Input: part model. Units: mm. Frame: model coordinates. Face numbers are marked on the shaded views. A direction names the side the tool comes from. Coordinates: 2 decimals unless noted, no trailing zeros. Order: outer loops, then holes, each group sorted by start corner. A loop starts at its lowest first (then second) coordinate and runs counter-clockwise, first axis right, second up. Notation, with made-up numbers: (-11.5, -33.75) -> (34.5, -33.75) arc R21 ccw to (34.5, -4.75) -> close; hole circle Ø10 at (15.5, -38). An arc over 180 degrees is marked (long way). Write each question's results on one line, items separated by ' | '.
```python
from build123d import *

# Parameters (mm, degrees)
BOSS_EXTRUDE1_DEPTH     = 57
SKETCH3_W               = 33
SKETCH3_H               = 9
SKETCH3_W_2             = 9
SKETCH3_H_2             = 15.5
CUT_EXTRUDE2_DEPTH      = 86.030876745
FILLET1_R               = 4
CUT_EXTRUDE3_DEPTH      = 86.030876745
CUT_EXTRUDE4_REACH      = 81.789
CUT_EXTRUDE5_DEPTH      = 3.5
SKETCH9_R               = 3.2
SKETCH10_R              = 2.8
CUT_EXTRUDE6_DEPTH      = 82.124903768
CUT_EXTRUDE6_DEPTH_BACK = 82.124903768
SKETCH11_R              = 2
SKETCH13_R              = 2
CUT_EXTRUDE7_DEPTH      = 20
SKETCH14_R              = 1.75
SKETCH14_R_2            = 5.5
BOSS_EXTRUDE2_DEPTH     = 10
BOSS_EXTRUDE3_DEPTH     = 30
SKETCH16_R              = 2.1
CUT_EXTRUDE8_DEPTH      = 3.4
SKETCH18_R              = 2.1
CUT_EXTRUDE9_DEPTH      = 9


with BuildPart() as part:
    # Sketch1 → Boss-Extrude1 (new body)
    with BuildSketch(Plane.XY):
        Polygon((0, 0), (0, -35), (19, -35), (19, -16), (52.5, -16), (52.5, 0), align=None)
    extrude(amount=BOSS_EXTRUDE1_DEPTH)

    # Sketch3 → Cut-Extrude2 (cut, through all)
    with BuildSketch(Plane.ZY):
        with Locations((28.5, -8)):
            Rectangle(SKETCH3_W, SKETCH3_H)
        with Locations((52.5, -27.25)):
            Rectangle(SKETCH3_W_2, SKETCH3_H_2)
    extrude(amount=-CUT_EXTRUDE2_DEPTH, mode=Mode.SUBTRACT)

    # Fillet1
    fillet1_edges = [part.edges().sort_by_distance(p)[0] for p in [
        (26.25, 0, 57),
        (9.5, -19.5, 57),
    ]]
    fillet(fillet1_edges, radius=FILLET1_R)

    # Sketch4 → Cut-Extrude3 (cut, through all)
    with BuildSketch(Plane(origin=(0, 0, 0), x_dir=(-1, 0, 0), z_dir=(0, 0, -1))):
        with BuildLine():
            Line((-0.01301942, -25.002808416), (-2.010278489, -25.107480328))
            ThreePointArc((-2.010278489, -25.107480328), (-16.998857714, -25.369106952), (-2.028539764, -26.153668071))
            Line((-2.028539764, -26.153668071), (-0.036150368, -26.327979556))
            ThreePointArc((-0.036150368, -26.327979556), (-3.081893028, -32.5041347), (-9.5, -35))
            Line((-9.5, -35), (0, -35))
            Line((0, -35), (0, -25.002053723))
            Line((0, -25.002053723), (-0.01301942, -25.002808416))
        make_face()
        with BuildLine():
            ThreePointArc((-9.5, -35), (-16.217514421, -32.217514421), (-19, -25.5))
            Line((-19, -25.5), (-19, -35))
            Line((-19, -35), (-9.5, -35))
        make_face()
    extrude(amount=-CUT_EXTRUDE3_DEPTH, mode=Mode.SUBTRACT)

    # Cut-Extrude4: up to this face of the body (flat: up to its plane)
    cut_extrude4_end = Plane(part.part.faces().sort_by_distance((26.25, -3.5, 28.5))[0])
    # Sketch5 → Cut-Extrude4 (cut, up to the picked face)
    with BuildSketch(Plane.XZ.offset(16), mode=Mode.PRIVATE) as cut_extrude4_sk1:
        with BuildLine():
            Line((47, 18.7), (36, 18.7))
            ThreePointArc((36, 18.7), (34.3, 17), (36, 15.3))
            Line((36, 15.3), (47, 15.3))
            ThreePointArc((47, 15.3), (48.7, 17), (47, 18.7))
        make_face()
    cut_extrude4_tool1 = split(extrude(cut_extrude4_sk1.sketch, amount=-CUT_EXTRUDE4_REACH, mode=Mode.PRIVATE), bisect_by=cut_extrude4_end, keep=Keep.BOTH, mode=Mode.PRIVATE)
    # Sketch5 → Cut-Extrude4 (cut, up to the picked face)
    with BuildSketch(Plane.XZ.offset(16), mode=Mode.PRIVATE) as cut_extrude4_sk2:
        with BuildLine():
            Line((40.5, 21), (49.5, 21))
            ThreePointArc((49.5, 21), (51.621320344, 20.121320344), (52.5, 18))
            Line((52.5, 18), (52.5, 57))
            Line((52.5, 57), (40.5, 57))
            Line((40.5, 57), (40.5, 21))
        make_face()
    cut_extrude4_tool2 = split(extrude(cut_extrude4_sk2.sketch, amount=-CUT_EXTRUDE4_REACH, mode=Mode.PRIVATE), bisect_by=cut_extrude4_end, keep=Keep.BOTH, mode=Mode.PRIVATE)
    add(cut_extrude4_tool1.solids().sort_by(Axis((41.5, -16, 17), (0, 1, 0)))[0], mode=Mode.SUBTRACT)
    add(cut_extrude4_tool2.solids().sort_by(Axis((46.523723, -16, 38.9169), (0, 1, 0)))[0], mode=Mode.SUBTRACT)

    # Sketch6 → Cut-Extrude5 (cut)
    with BuildSketch(Plane(origin=(0, 0, 0), x_dir=(1, 0, 0), z_dir=(0, 1, 0))):
        with BuildLine():
            Line((10, -12), (21, -12))
            ThreePointArc((21, -12), (22.414213562, -12.585786438), (23, -14))
            Line((23, -14), (23, -43))
            ThreePointArc((23, -43), (22.414213562, -44.414213562), (21, -45))
            Line((21, -45), (10, -45))
            ThreePointArc((10, -45), (8.585786438, -44.414213562), (8, -43))
            Line((8, -43), (8, -14))
            ThreePointArc((8, -14), (8.585786438, -12.585786438), (10, -12))
        make_face()
        with BuildLine():
            Line((43.5, -11.968626967), (52.5, -11.968626967))
            Line((52.5, -11.968626967), (52.5, -56.968626967))
            Line((52.5, -56.968626967), (40.5, -56.968626967))
            Line((40.5, -56.968626967), (40.5, -14.968626967))
            ThreePointArc((40.5, -14.968626967), (41.378679656, -12.847306623), (43.5, -11.968626967))
        make_face()
    extrude(amount=-CUT_EXTRUDE5_DEPTH, mode=Mode.SUBTRACT)

    # Sketch9 → Loft1 section 0
    with BuildSketch(Plane.XZ.offset(3.5)):
        with Locations((27, 28.5)):
            Circle(SKETCH9_R)
    # Sketch10 → Loft1 section 1
    with BuildSketch(Plane(origin=(0, -5, 0), x_dir=(-1, 0, 0), z_dir=(0, -1, 0))):
        with Locations((-27, -28.5)):
            Circle(SKETCH10_R)
    loft1 = loft()

    # Mirror2: Loft1 across plane
    add(loft1.mirror(Plane(origin=(0, -8, 0), x_dir=(0, 0, 1), z_dir=(0, -1, 0))))

    # Sketch11 → Cut-Extrude6 (cut, two sides: drawn at the far end of the back side and taken through both)
    with BuildSketch(Plane(origin=(0, -11, 0), x_dir=(1, 0, 0), z_dir=(0, 1, 0)).offset(-CUT_EXTRUDE6_DEPTH_BACK)):
        with Locations(Location((27, -28.5, 0), (0, 0, 270))):
            Circle(SKETCH11_R)
    extrude(amount=CUT_EXTRUDE6_DEPTH + CUT_EXTRUDE6_DEPTH_BACK, mode=Mode.SUBTRACT)

    # Sketch13 → Cut-Extrude7 (cut)
    with BuildSketch(Plane(origin=(52.5, 0, 0), x_dir=(0, 0, -1), z_dir=(1, 0, 0))):
        with Locations((-6, -8)):
            Circle(SKETCH13_R)
        with Locations((-51, -8)):
            Circle(SKETCH13_R)
    extrude(amount=-CUT_EXTRUDE7_DEPTH, mode=Mode.SUBTRACT)

    # Sketch14 → Boss-Extrude2 (add)
    # profile 1 of 2: a face of its own
    with BuildSketch(Plane(origin=(0, 0, 0), x_dir=(-1, 0, 0), z_dir=(0, 0, -1))):
        with BuildLine():
            ThreePointArc((-19, -19.954731747), (-20.721825407, -17.721825407), (-22.954731747, -16))
            Line((-22.954731747, -16), (-34.045268253, -16))
            ThreePointArc((-34.045268253, -16), (-35.581002842, -33.917802489), (-18.190789474, -29.336688458))
            ThreePointArc((-18.190789474, -29.336688458), (-18.795496221, -27.460548393), (-19, -25.5))
            Line((-19, -25.5), (-19, -19.954731747))
        make_face()
        with Locations((-33.425291803, -31.804086029)):
            Circle(SKETCH14_R, mode=Mode.SUBTRACT)
        with Locations((-22.195913971, -30.425291803)):
            Circle(SKETCH14_R, mode=Mode.SUBTRACT)
        with Locations((-34.804086029, -20.574708197)):
            Circle(SKETCH14_R, mode=Mode.SUBTRACT)
        with Locations((-28.5, -25.5)):
            Circle(SKETCH14_R_2, mode=Mode.SUBTRACT)
        with Locations((-23.574708197, -19.195913971)):
            Circle(SKETCH14_R, mode=Mode.SUBTRACT)
    # profile 2 of 2: a face of its own
    with BuildSketch(Plane(origin=(0, 0, 0), x_dir=(-1, 0, 0), z_dir=(0, 0, -1))):
        with BuildLine():
            Line((-19, -16), (-22.954731747, -16))
            ThreePointArc((-22.954731747, -16), (-20.721825407, -17.721825407), (-19, -19.954731747))
            Line((-19, -19.954731747), (-19, -16))
        make_face()
    extrude(amount=-BOSS_EXTRUDE2_DEPTH)

    # Sketch15 → Boss-Extrude3 (add)
    with BuildSketch(Plane.ZY):
        with BuildLine():
            Line((53, -19.5), (48, -19.5))
            Line((48, -19.5), (48, 0))
            Line((48, 0), (53, 0))
            ThreePointArc((53, 0), (55.828427125, -1.171572875), (57, -4))
            Line((57, -4), (57, -15.5))
            ThreePointArc((57, -15.5), (55.828427125, -18.328427125), (53, -19.5))
        make_face()
    extrude(amount=BOSS_EXTRUDE3_DEPTH)

    # Sketch16 → Cut-Extrude8 (cut)
    with BuildSketch(Plane.XY.offset(55)):
        Polygon((-30, -13.35), (-22.921539031, -13.35), (-20.843078062, -9.75), (-22.921539031, -6.15), (-30, -6.15), align=None)
        with Locations((-26, -9.75)):
            Circle(SKETCH16_R, mode=Mode.SUBTRACT)
    extrude(amount=-CUT_EXTRUDE8_DEPTH, mode=Mode.SUBTRACT)

    # Sketch18 → Cut-Extrude9 (cut)
    with BuildSketch(Plane.XY.offset(57)):
        with Locations((-26, -9.75)):
            Circle(SKETCH18_R)
    extrude(amount=-CUT_EXTRUDE9_DEPTH, mode=Mode.SUBTRACT)


solid = part.part
```
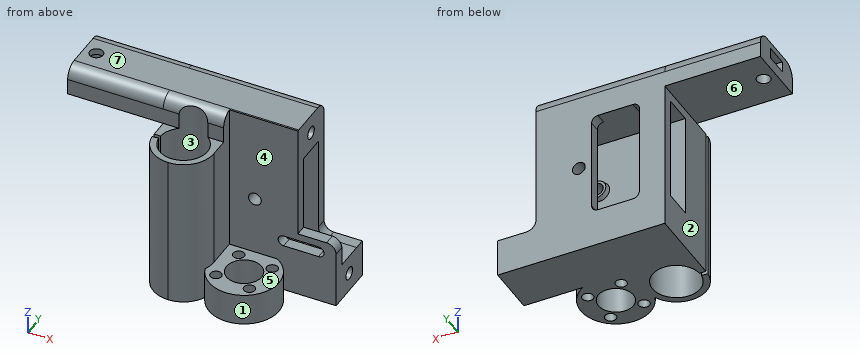
(1) Line query: line 1 along Z through (x, y) = (37, -4); line 2 along Y through (x, z) = (33.5, 41); line 3 along Z through (x, y) = (28, -12). Output: solid intervals per line, ascending. Write a range as from..to.
Return value:
line 1: 0..12, 45..57 | line 2: -16..-12.5, -3.5..0 | line 3: 0..12, 25.6..26.77, 30.23..31.4, 45..57
(2) Cut plane A-A, the plane z = 17. Count the separate pieces of the cut face and the enclosed holes in it, plus the area to 3 significant figures.
Return value:
separate pieces: 4 | enclosed holes: 0 | area: 366 mm2
(3) Pin query (flat end, axial travel): P1, Ø1.5, axis at x = 12.5, z = 19.5, coming from the +Y side; P2, Ø6.5, axis at x = -26, y = -9.75, coming from the -Z side; P3, Ø1, axis at x = 44.5, y = -14.5, coming from the +Z side; P4, Ø4, axis at y = -9, z = 34.5, coming from the +X side. Return the tip coordinate at first contact, or that it passes through.
Return value:
P1: y = -12.5 | P2: z = 48 | P3: z = 21 | P4: through
(4) Reachability of the marked faces 5, 6 and 7 from +Z, -Z, +X, -X, +Y, -Y: full face, straight path, thin tool, end or side. Return the list, or none.
Return value:
face 5: +Z, +X, -Y | face 6: -Z, -X, +Y, -Y | face 7: +Z, +X, -X, +Y, -Y
(5) Cut plane C-C, the plane x = -8.5. Return loops of the section in (y, z).
Return value:
outline: (-19.5, 48) -> (0, 48) -> (0, 53) arc R4 ccw to (-4, 57) -> (-15.5, 57) arc R4 ccw to (-19.5, 53) -> close
(6) Mould query, pull axis X, two halves, no side actions, for the marked faces 1, 2, 3 and 4. Classes: +X half, -X half, draft (parallel to the pull), parting line (faces both ways), or undercut.
Return value:
face 1: undercut | face 2: -X half | face 3: undercut | face 4: draft
